For this review, use the dimensioned drawing (mm, ordinates from the lowest corner) and the shaded views. Round coordinates to 2 decimals unless told otherwise and drop trailing zeros. Order: outer loops, then holes, each group sorted by start corner. A loop starts at its lowest first (then second) coordinate and runs counter-clockwise, first axis right, second up. Notation, with made-up numbers: (-8, 64) - (42, 64) arc R25 ccw to (42, 84) - close; hole circle Ø3 at (-16, 86). An arc over 180 degrees is marked (long way). Write each question's results on one line, items separated by ' | '. Start each with the question number.
(1) Take a section at A-A, the plane x = 30. Give the boundary of the cut face in (y, z).
(2) Insertion check: pin 1 Ø3 at (x, z) = (50, 50) entering from -Y; pin 2 Ø1 at (x, y) = (7.5, 3.5) entering from +Z. Each pin has a flat end and moves straight along its axis. Give the tip position at first contact, or say it passes through.
(3) Take a section at D-D, the plane z = 50. Give the boundary of the cut face in (x, y).
(4) Take a section at B-B, the plane z = 70. Give the boundary of the cut face in (x, y).
(5) Take a section at C-C, the plane y = 3. Give the boundary of the cut face in (x, z).
(6) For L1, parallel to Z at x = 30, y = 2.6; L2, parallel to Z at x = 50, y = 1.8; L3, parallel to Z at x = 12, y = 3.45, list the stretches that pass through material, from the lowest coordinate up. Write a range as from..to.
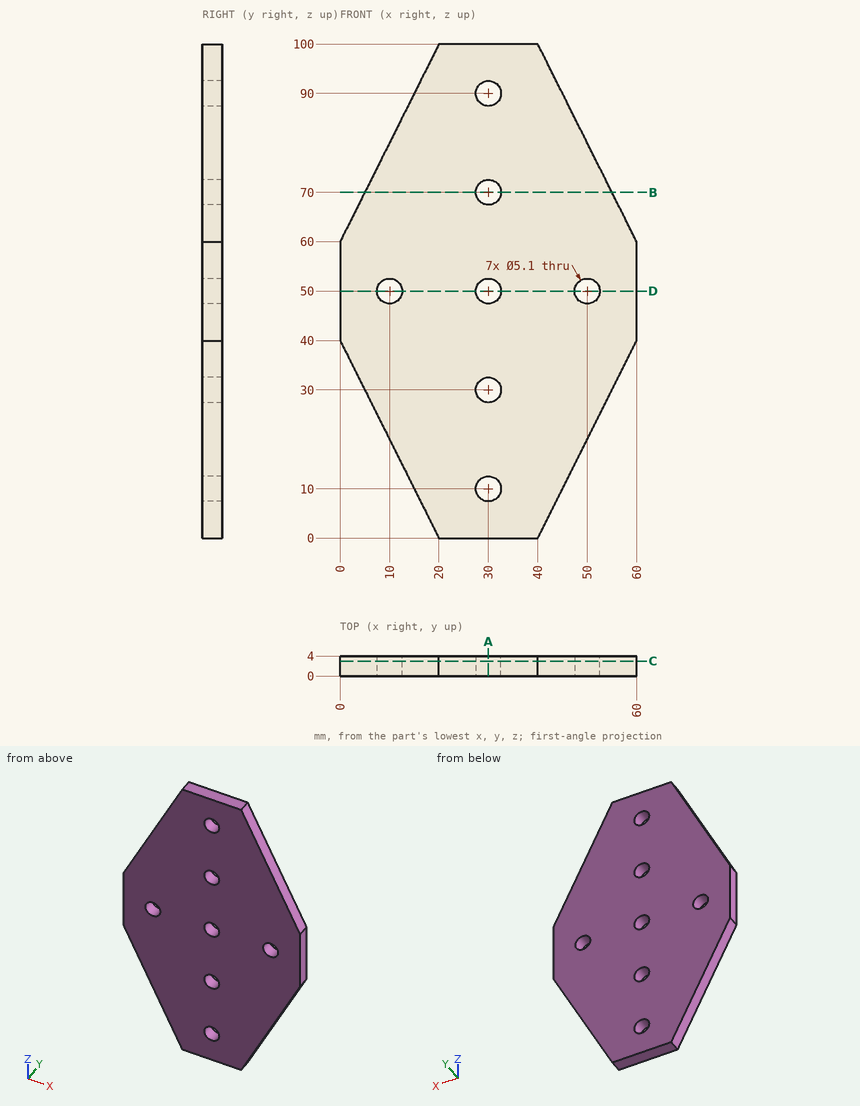
Results below:
1) outline: (0, 0) - (4, 0) - (4, 7.45) - (0, 7.45) - close; (0, 12.55) - (4, 12.55) - (4, 27.45) - (0, 27.45) - close; (0, 32.55) - (4, 32.55) - (4, 47.45) - (0, 47.45) - close; (0, 52.55) - (4, 52.55) - (4, 67.45) - (0, 67.45) - close; (0, 72.55) - (4, 72.55) - (4, 87.45) - (0, 87.45) - close; (0, 92.55) - (4, 92.55) - (4, 100) - (0, 100) - close
2) pin 1: passes through | pin 2: stops at z = 76
3) outline: (0, 0) - (7.45, 0) - (7.45, 4) - (0, 4) - close; (12.55, 0) - (27.45, 0) - (27.45, 4) - (12.55, 4) - close; (32.55, 0) - (47.45, 0) - (47.45, 4) - (32.55, 4) - close; (52.55, 0) - (60, 0) - (60, 4) - (52.55, 4) - close
4) outline: (5, 0) - (27.45, 0) - (27.45, 4) - (5, 4) - close; (32.55, 0) - (55, 0) - (55, 4) - (32.55, 4) - close
5) outline: (0, 40) - (20, 0) - (40, 0) - (60, 40) - (60, 60) - (40, 100) - (20, 100) - (0, 60) - close; hole circle Ø5.1 at (10, 50); hole circle Ø5.1 at (30, 10); hole circle Ø5.1 at (30, 30); hole circle Ø5.1 at (30, 50); hole circle Ø5.1 at (30, 70); hole circle Ø5.1 at (30, 90); hole circle Ø5.1 at (50, 50)
6) L1: z = 0..7.45, 12.55..27.45, 32.55..47.45, 52.55..67.45, 72.55..87.45, 92.55..100 | L2: z = 20..47.45, 52.55..80 | L3: z = 16..48.42, 51.58..84
